```python
from build123d import *

# Parameters (mm, degrees)
BOSS_EXTRU_1_DEPTH = 25
ESQUISSE2_R        = 2
BOSS_EXTRU_2_DEPTH = 4.5
ESQUISSE4_R        = 2
BOSS_EXTRU_3_DEPTH = 4.5


with BuildPart() as part:
    # Esquisse1 → Boss.-Extru.1 (new body)
    with BuildSketch(Plane.XY):
        Polygon((0, 0), (195, 0), (195, -38), (185, -38), (175, -28), (185, -28), (185, -10), (10, -10), (10, -28), (20, -28), (10, -38), (0, -38), align=None)
    extrude(amount=BOSS_EXTRU_1_DEPTH)

    # Esquisse2 → Boss.-Extru.2 (add)
    with BuildSketch(Plane.XY.offset(25)):
        with BuildLine():
            Line((97.5, 0), (87.5, 0))
            add(Edge.make_bspline(
                [(93, 12), (93.473540625, 4.530107825), (87.5, 0)],
                knots=[0, 0, 0, 1, 1, 1], degree=2))
            ThreePointArc((93, 12), (97.5, 16.5), (102, 12))
            add(Edge.make_bspline(
                [(102, 12), (101.526459375, 4.530107825), (107.5, 0)],
                knots=[0, 0, 0, 1, 1, 1], degree=2))
            Line((107.5, 0), (97.5, 0))
        make_face()
        with Locations((97.5, 12)):
            Circle(ESQUISSE2_R, mode=Mode.SUBTRACT)
    extrude(amount=-BOSS_EXTRU_2_DEPTH)

    # Esquisse4 → Boss.-Extru.3 (add)
    with BuildSketch(Plane(origin=(0, 0, 0), x_dir=(-1, 0, 0), z_dir=(0, 0, -1))):
        with BuildLine():
            Line((-97.5, 0), (-107.5, 0))
            add(Edge.make_bspline(
                [(-102, 12), (-101.527789756, 4.527189734), (-107.5, 0)],
                knots=[0, 0, 0, 1, 1, 1], degree=2))
            ThreePointArc((-102, 12), (-97.5, 16.5), (-93, 12))
            add(Edge.make_bspline(
                [(-93, 12), (-93.472210244, 4.527189734), (-87.5, 0)],
                knots=[0, 0, 0, 1, 1, 1], degree=2))
            Line((-87.5, 0), (-97.5, 0))
        make_face()
        with Locations((-97.5, 12)):
            Circle(ESQUISSE4_R, mode=Mode.SUBTRACT)
    extrude(amount=-BOSS_EXTRU_3_DEPTH)


solid = part.part
```
Geometry: final body of the model. Coordinates: model frame, mm. A direction names the side the tool comes from. Round coordinates to 2 decimals unless told otherwise and drop trailing zeros. Order: outer loops, then holes, each group sorted by start corner. A loop starts at its lowest first (then second) coordinate and runs counter-clockwise, first axis right, second up. Notation, with made-up numbers: M -31.5,81 L 5.5,81 A8 cw 5.5,94 Z; hole C 36,19 d6. An arc over 180 degrees is marked long. One line per item, written item: value.
(1) Cut plane B-B (x = 97.5). Return the cut outline in (y, z).
Result sheet:
outline: M -10,0 L 10,0 L 10,4.5 L 0,4.5 L 0,20.5 L 10,20.5 L 10,25 L -10,25 Z; M 14,0 L 16.5,0 L 16.5,4.5 L 14,4.5 Z; M 14,20.5 L 16.5,20.5 L 16.5,25 L 14,25 Z
(2) Cut plane D-D (x = 179.5). Return the cut outline in (y, z).
Result sheet:
outline: M -32.5,0 L -28,0 L -28,25 L -32.5,25 Z; M -10,0 L 0,0 L 0,25 L -10,25 Z
(3) Cut plane C-C (z = 18.25). Return the cut outline in (x, y).
Result sheet:
outline: M 0,-38 L 10,-38 L 20,-28 L 10,-28 L 10,-10 L 185,-10 L 185,-28 L 175,-28 L 185,-38 L 195,-38 L 195,0 L 0,0 Z
(4) Pull-direction query (X, two-part tool) for faces 5 (the flat face through (195, -19, 12)), 6 (the flat face through (15, -33, 12)), 7 (the flat face through (5, -38, 12)); classes: pulls with the +X half, pulls with the -X half, needs draft (parallel to the pull), parting line crosses it, or undercut.
Result sheet:
face 5: pulls with the +X half
face 6: undercut
face 7: needs draft
(5) Pin query (flat end, axial travel): P1, Ø1.5, axis at x = 146, z = 21.5, coming from the +Y side; P2, Ø12.5, axis at x = 56.5, z = 7, coming from the -Y side; P3, Ø6, axis at y = 7.5, z = 22, coming from the +X side. Return the tip coordinate at first contact, or that it passes through.
Result sheet:
P1: y = 0
P2: y = -10
P3: x = 103.52
(6) Cut plane A-A (x = 17). Return the cut outline in (y, z).
Result sheet:
outline: M -31,0 L -28,0 L -28,25 L -31,25 Z; M -10,0 L 0,0 L 0,25 L -10,25 Z
(7) Reachability of faces 1 (the flat face through (97, 7, 20.5)), 2 (the flat face through (180, -28, 12)), 3 (the flat face through (98, -7, 0)), 4 (the flat face through (180, -33, 12)) from +Z, -Z, +X, -X, +Y, -Y: full face, straight path, thin tool, end or side. Return the list, or none.
Result sheet:
face 1: +X, -X, +Y
face 2: +Z, -Z
face 3: -Z, +X, -X, +Y, -Y
face 4: +Z, -Z, -Y
(8) Line query: probe 1 along Y at (x, z) = (97.5, 2.7); probe 2 along X at (y, z) = (-16, 23); probe 3 along Y at (x, z) = (136, 5.75). Output: solid intervals per line, ascending. Write a range as [from, to].
Result sheet:
probe 1: [-10, 10], [14, 16.5]
probe 2: [0, 10], [185, 195]
probe 3: [-10, 0]
